Can you work these out from the model? Positions are in its coordinate system, mm. A direction names the side the tool comes from. Give positions to 0.01 mm unless a question says otherwise; leave off trailing zeros. Loops run counter-clockwise (first coordinate to the right, second up) from the corner with the lowest first, then second, coordinate; pieces in that order, holes last. Notation, with made-up numbers: (2.5, -36.75) -> (15.5, -36.75) arc R27 ccw to (15.5, -5.75) -> close; hole circle Ø5 at (58.25, 57). An arc over 180 degrees is marked (long way). Return JSON: item names as keys, results as strings. Group by question number.
Q1. Which directions (+Z, -Z, +X, -X, +Y, -Y) give clear straight access to the entire face, cutting with the end or side of a thin tool? Please do faces 5 (the cylindrical face through (0.224, 24.867, 219.3)), 6 (the cylindrical face through (-29.97, 1.32, 274.93)), 7 (the cylindrical face through (-60.225, 9.704, 59.16)), 8 (the flat face through (21, 0, 170)).
Q2. Suppose I cut it at C-C, the plane z = 60. Please give me the cut outline in (x, y), and give its area (3 significant figures).
Q3. I need wall thicknesses on line 1 along Y through (x, z) = (-45.5, 60); line 2 along Z through (x, y) = (-22, 1); line 3 along Y through (x, z) = (0, 287). Which ranges of each line are inside material? Lowest first, please. Write a range as [from, to].
Q4. Thinking about a two-plate mould opening in Z: for faces 1 (the cylindrical face through (60.695, 0.653, 59.16)), 2 (the cylindrical face through (-51.14, -34.862, 48.944)), 3 (the cylindrical face through (-0.224, -24.867, 219.3)), 4 (the conical face through (54.514, -0.613, 126.181)), which applies, pulls with the +Z half, pulls with the -Z half, needs draft (parallel to the pull), parting line crosses it, or undercut?
Q5. Suppose I cut it at B-B, the plane x = -24. Please give me the cut outline in (y, z).
Q6. Will these pins go through, and if not, where does the flat tip stop? pin 1 (15 mm diameter, centred on y = -49.5, z = 64.5, fed in from -X); pin 2 (8 mm diameter, centred on x = -32, z = 121.5, fed in from -Y); pin 3 (21.5 mm diameter, centred on x = -8.5, y = -53.5, fed in from +Z).
```python
from build123d import *

# Parameters (mm, degrees)
BOSS_EXTRUDE1_DEPTH = 120
BOSS_EXTRUDE2_DEPTH = 10
BOSS_EXTRUDE2_TAPER = 45
SKETCH3_R           = 35
BOSS_EXTRUDE3_DEPTH = 10
SKETCH4_R           = 32.5
BOSS_EXTRUDE4_DEPTH = 30
BOSS_EXTRUDE5_DEPTH = 100
SKETCH6_R           = 30
BOSS_EXTRUDE6_DEPTH = 10
SKETCH7_R           = 28
BOSS_EXTRUDE7_DEPTH = 11
SKETCH8_R           = 40
BOSS_EXTRUDE8_DEPTH = 11
BOSS_EXTRUDE9_DEPTH = 55
SKETCH10_R          = 15
CUT_EXTRUDE1_DEPTH  = 11
SKETCH11_R          = 15
CUT_EXTRUDE2_DEPTH  = 20


with BuildPart() as part:
    # Sketch1 → Boss-Extrude1 (new body)
    with BuildSketch(Plane.XY):
        with BuildLine():
            Line((-50, 45), (50, 45))
            ThreePointArc((50, 45), (60.697144503, 0), (50, -45))
            Line((50, -45), (-50, -45))
            ThreePointArc((-50, -45), (-60.697144503, 0), (-50, 45))
        make_face()
    extrude(amount=BOSS_EXTRUDE1_DEPTH)

    # Sketch2 → Boss-Extrude2 (add)
    with BuildSketch(Plane.XY.offset(120)):
        with BuildLine():
            Line((-50, -45), (50, -45))
            ThreePointArc((50, -45), (60.697144503, 0), (50, 45))
            Line((50, 45), (-50, 45))
            ThreePointArc((-50, 45), (-60.697144503, 0), (-50, -45))
        make_face()
    extrude(amount=BOSS_EXTRUDE2_DEPTH, taper=BOSS_EXTRUDE2_TAPER)

    # Sketch3 → Boss-Extrude3 (add)
    with BuildSketch(Plane.XY.offset(130)):
        Circle(SKETCH3_R)
    extrude(amount=BOSS_EXTRUDE3_DEPTH)

    # Sketch4 → Boss-Extrude4 (add)
    with BuildSketch(Plane.XY.offset(140)):
        Circle(SKETCH4_R)
    extrude(amount=BOSS_EXTRUDE4_DEPTH)

    # Sketch5 → Boss-Extrude5 (add)
    with BuildSketch(Plane.XY.offset(170)):
        with BuildLine():
            Line((-15, 20), (-15, -20))
            ThreePointArc((-15, -20), (0, -24.86796738), (15, -20))
            Line((15, -20), (15, 20))
            ThreePointArc((15, 20), (0, 24.86796738), (-15, 20))
        make_face()
    extrude(amount=BOSS_EXTRUDE5_DEPTH)

    # Sketch6 → Boss-Extrude6 (add)
    with BuildSketch(Plane.XY.offset(270)):
        Circle(SKETCH6_R)
    extrude(amount=BOSS_EXTRUDE6_DEPTH)

    # Sketch7 → Boss-Extrude7 (add)
    with BuildSketch(Plane.XY.offset(280)):
        Circle(SKETCH7_R)
    extrude(amount=BOSS_EXTRUDE7_DEPTH)

    # Sketch8 → Boss-Extrude8 (add, symmetric)
    with BuildSketch(Plane.ZY.offset(50)):
        with Locations((60, -45)):
            Circle(SKETCH8_R)
    extrude(amount=BOSS_EXTRUDE8_DEPTH, both=True)

    # Sketch9 → Boss-Extrude9 (add)
    with BuildSketch(Plane(origin=(-39, 0, 0), x_dir=(0, 0, -1), z_dir=(1, 0, 0))):
        with BuildLine():
            Line((-85, -45), (-35, -45))
            Line((-35, -45), (-35, -72))
            ThreePointArc((-35, -72), (-60, -76.80636081), (-85, -72))
            Line((-85, -72), (-85, -45))
        make_face()
    extrude(amount=BOSS_EXTRUDE9_DEPTH)

    # Sketch10 → Cut-Extrude1 (cut)
    with BuildSketch(Plane.XY.offset(291)):
        Circle(SKETCH10_R)
    extrude(amount=-CUT_EXTRUDE1_DEPTH, mode=Mode.SUBTRACT)

    # Sketch11 → Cut-Extrude2 (cut)
    with BuildSketch(Plane.ZY.offset(61)):
        with Locations((60, -45)):
            Circle(SKETCH11_R)
    extrude(amount=-CUT_EXTRUDE2_DEPTH, mode=Mode.SUBTRACT)


solid = part.part
```
Ans:
{
 "1": {"face 5": "+Y", "face 6": "+Z", "face 7": "-X", "face 8": "none"},
 "2": {"outline": "(-61, -85) -> (-39, -85) -> (-39, -76.81) -> (16, -76.81) -> (16, -45) -> (50, -45) arc R100 ccw to (50, 45) -> (-50, 45) arc R100 ccw to (-60.57, -5) -> (-61, -5) -> (-61, -30) -> (-41, -30) -> (-41, -60) -> (-61, -60) -> close", "area": "12,500 mm^2"},
 "3": {"line 1": "y = [-85, -60], [-30, 45]", "line 2": "z = [0, 170], [270, 291]", "line 3": "y = [-28, -15], [15, 28]"},
 "4": {"face 1": "needs draft", "face 2": "undercut", "face 3": "undercut", "face 4": "pulls with the +Z half"},
 "5": {"outline": "(-72, 35) -> (-45, 35) -> (-45, 0) -> (45, 0) -> (45, 120) -> (35, 130) -> (25.48, 130) -> (25.48, 140) -> (21.91, 140) -> (21.91, 170) -> (-21.91, 170) -> (-21.91, 140) -> (-25.48, 140) -> (-25.48, 130) -> (-35, 130) -> (-45, 120) -> (-45, 85) -> (-72, 85) arc R67.42 ccw to start; (-18, 270) -> (18, 270) -> (18, 280) -> (14.42, 280) -> (14.42, 291) -> (-14.42, 291) -> (-14.42, 280) -> (-18, 280) -> close"},
 "6": {"pin 1": "stops at x = -41", "pin 2": "stops at y = -45", "pin 3": "stops at z = 122.25"}
}
